from build123d import *

# Parameters (mm, degrees)
CROQUIS1_W              = 31
CROQUIS1_H              = 70
CROQUIS1_W_2            = 27
CROQUIS1_H_2            = 66
SALIENTE_EXTRUIR1_DEPTH = 40
CROQUIS4_W              = 40.3
CROQUIS4_H              = 20.15
CROQUIS4_R              = 2.15
SALIENTE_EXTRUIR2_DEPTH = 31
CROQUIS5_W              = 27
CROQUIS5_H              = 40.3
CORTAR_EXTRUIR2_DEPTH   = 40
CROQUIS6_W              = 31
CROQUIS6_H              = 70
SALIENTE_EXTRUIR3_DEPTH = 3


with BuildPart() as part:
    # Croquis1 → Saliente-Extruir1 (new body)
    with BuildSketch(Plane(origin=(0, 0, 0), x_dir=(1, 0, 0), z_dir=(0, 1, 0))):
        Rectangle(CROQUIS1_W, CROQUIS1_H)
        Rectangle(CROQUIS1_W_2, CROQUIS1_H_2, mode=Mode.SUBTRACT)
    extrude(amount=SALIENTE_EXTRUIR1_DEPTH)

    # Croquis4 → Saliente-Extruir2 (add, through all)
    with BuildSketch(Plane(origin=(15.5, 0, 0), x_dir=(0, 0, -1), z_dir=(1, 0, 0))):
        with Locations((0, 50.075)):
            Rectangle(CROQUIS4_W, CROQUIS4_H)
        with Locations((-16, 56)):
            Circle(CROQUIS4_R, mode=Mode.SUBTRACT)
        with Locations((16, 56)):
            Circle(CROQUIS4_R, mode=Mode.SUBTRACT)
    extrude(amount=-SALIENTE_EXTRUIR2_DEPTH)

    # Croquis5 → Cortar-Extruir2 (cut)
    with BuildSketch(Plane(origin=(0, 60.15, 0), x_dir=(1, 0, 0), z_dir=(0, 1, 0))):
        Rectangle(CROQUIS5_W, CROQUIS5_H)
    extrude(amount=-CORTAR_EXTRUIR2_DEPTH, mode=Mode.SUBTRACT)

    # Croquis6 → Saliente-Extruir3 (add)
    with BuildSketch(Plane.XZ):
        Rectangle(CROQUIS6_W, CROQUIS6_H)
    extrude(amount=-SALIENTE_EXTRUIR3_DEPTH)


solid = part.part
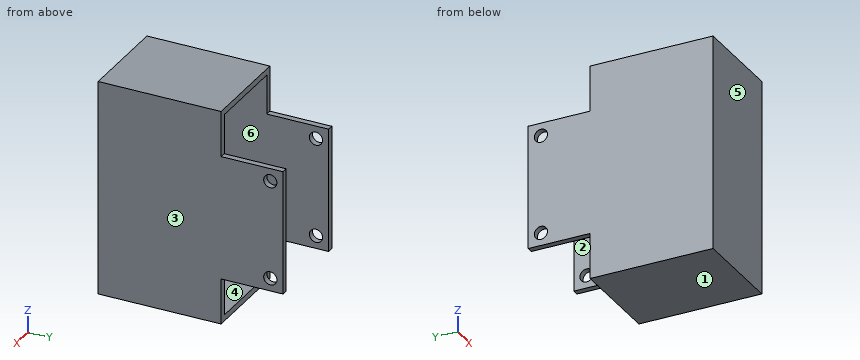
The model under review builds one solid part; all positions refer to its coordinate system, in mm. Face numbers are marked on the shaded views. A direction names the side the tool comes from. Round coordinates to 2 decimals unless told otherwise and drop trailing zeros. Write each loop counter-clockwise with the first axis right and the second up, starting at its lowest first coordinate (ties: lowest second). Pieces come first, ordered by that corner, then holes. Notation, with made-up numbers: (76.25, 51.25) -> (91.25, 51.25) arc R29 cw to (91.25, 73.25) -> close; hole circle Ø8 at (29, -24.75). An arc over 180 degrees is marked (long way). Answer as a JSON object with one key per item and string values.
1. Machinability: for the marked faces 5 and 6, which of the approach directions +Z, -Z, +X, -X, +Y, -Y give a long, thin tool a straight path to every point of the face, cutting with its end or side? Answer none if there is none.
Results found:
{"face 5": "+Z, -Z, +X, -X, -Y", "face 6": "+Y"}
2. We need section B-B on y = 52.5. State the section outline as (x, z) points.
Results found:
{"outline": "(-15.5, -20.15) -> (-13.5, -20.15) -> (-13.5, 20.15) -> (-15.5, 20.15) -> close; (13.5, -20.15) -> (15.5, -20.15) -> (15.5, 20.15) -> (13.5, 20.15) -> close"}
3. Clearance check with flat-ended pins moving along their axes: pin 1 (4 mm diameter, centred on x = -0.5, z = 25, fed in from +Y); pin 2 (1.6 mm diameter, centred on x = 15, y = 53, fed in from +Z); pin 3 (16.5 mm diameter, centred on x = 1.5, z = -26.5, fed in from +Y). State where each tip first meets the part, or that it passes through.
Results found:
{"pin 1": "stops at y = 3", "pin 2": "stops at z = 20.15", "pin 3": "stops at y = 40"}
4. The part is to be moulded in two halves that separate along Z. For the marked faces 1, 2, 3 and 4, say which applies: pulls with the +Z half, pulls with the -Z half, needs draft (parallel to the pull), parting line crosses it, or undercut.
Results found:
{"face 1": "pulls with the -Z half", "face 2": "undercut", "face 3": "needs draft", "face 4": "undercut"}
5. To check wall thickness, follow line 1 along Z through (x, y) = (12, 38); line 2 along X through (y, z) = (24.5, -19.5); line 3 along Y through (x, z) = (-14.85, 16). State the ranges of each line that lie inside material, in increasing order.
Results found:
{"line 1": "z = -35 to -33, 33 to 35", "line 2": "x = -15.5 to -13.5, 13.5 to 15.5", "line 3": "y = 0 to 53.85, 58.15 to 60.15"}
6. We need section A-A on z = 16. State the section outline as (x, y) points.
Results found:
{"outline": "(-15.5, 0) -> (15.5, 0) -> (15.5, 53.85) -> (13.5, 53.85) -> (13.5, 3) -> (-13.5, 3) -> (-13.5, 53.85) -> (-15.5, 53.85) -> close; (-15.5, 58.15) -> (-13.5, 58.15) -> (-13.5, 60.15) -> (-15.5, 60.15) -> close; (13.5, 58.15) -> (15.5, 58.15) -> (15.5, 60.15) -> (13.5, 60.15) -> close"}
7. We need section D-D on x = -1. State the section outline as (y, z) points, and give its area (3 significant figures).
Results found:
{"outline": "(0, -35) -> (40, -35) -> (40, -33) -> (3, -33) -> (3, 33) -> (40, 33) -> (40, 35) -> (0, 35) -> close", "area": "358 mm^2"}
8. We need section C-C on y = 22. State the section outline as (x, z) points, and give its area (3 significant figures).
Results found:
{"outline": "(-15.5, -35) -> (15.5, -35) -> (15.5, 35) -> (-15.5, 35) -> close; hole (-13.5, -33) -> (13.5, -33) -> (13.5, 33) -> (-13.5, 33) -> close", "area": "388 mm^2"}
